```python
from build123d import *

# Parameters (mm, degrees)
F0_R     = 30.348446
F0_R_2   = 27.203675
F1_DEPTH = 15
F2_R     = 53.512853
F3_DEPTH = 18
F4_DEPTH = 81.4
F5_SIZE  = 5


with BuildPart() as f1:
    # F0 (on Top) → F1 (new body)
    with BuildSketch(Plane.XY):
        Circle(F0_R)
        Circle(F0_R_2, mode=Mode.SUBTRACT)
    extrude(amount=F1_DEPTH)

    # F2 (on face) → F3 (join)
    with BuildSketch(Plane.XY.offset(15)):
        Circle(F2_R)
    extrude(amount=F3_DEPTH)

    # F0 (on Top) → F4 (cut)
    with BuildSketch(Plane.XY):
        Circle(F0_R_2)
    extrude(amount=F4_DEPTH, mode=Mode.SUBTRACT)

    # F5
    f5_edges = [f1.edges().sort_by_distance(p)[0] for p in [
        (-53.512853, 0, 15),
    ]]
    chamfer(f5_edges, length=F5_SIZE)


solid = f1.part
```
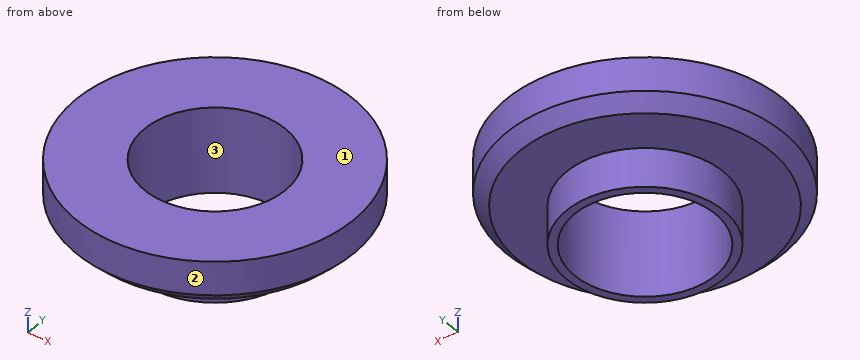
Geometry: final body of the model. Coordinates: model frame, mm. Face numbers are marked on the shaded views. Round coordinates to 2 decimals unless told otherwise and drop trailing zeros. Write each loop counter-clockwise with the first axis right and the second up, starting at its lowest first coordinate (ties: lowest second). Pieces come first, ordered by that corner, then holes. Notation, with made-up numbers: (-28, -33.75) -> (8, -33.75) arc R12 ccw to (8, -13.75) -> close; hole circle Ø1 at (89.25, 33.25). An arc over 180 degrees is marked (long way). Return JSON: item names as keys, results as strings.
Q1. Mould query, pull axis Y, two halves, no side actions, for the marked faces 1, 2 and 3. Classes: +Y half, -Y half, draft (parallel to the pull), parting line (faces both ways), or undercut.
From the geometry:
{"face 1": "draft", "face 2": "parting line", "face 3": "undercut"}
Q2. Section A-A on x = 0. Return the cut outline in (y, z).
From the geometry:
{"outline": "(-53.51, 20) -> (-48.51, 15) -> (-30.35, 15) -> (-30.35, 0) -> (-27.2, 0) -> (-27.2, 33) -> (-53.51, 33) -> close; (27.2, 0) -> (30.35, 0) -> (30.35, 15) -> (48.51, 15) -> (53.51, 20) -> (53.51, 33) -> (27.2, 33) -> close"}
Q3. Ray query, line 1 (Y direction, x = 0, z = 26); line 2 (Z direction, x = -8, y = -42.5); line 3 (X direction, y = 11.5, z = 10). Return the intervals inside material, ascending.
From the geometry:
{"line 1": "-53.51 to -27.2, 27.2 to 53.51", "line 2": "15 to 33", "line 3": "-28.09 to -24.65, 24.65 to 28.09"}
Q4. Section C-C on z = 11. Return the cut outline in (x, y), and give its area (3 significant figures).
From the geometry:
{"outline": "circle Ø60.7 at (0, 0); hole circle Ø54.41 at (0, 0)", "area": "569 mm2"}
Q5. First-contact query: pin 1 Ø5 at (x, z) = (-42, 28) entering from -Y; pin 2 Ø1.5 at (x, z) = (41, 24) entering from -Y; pin 3 Ø12 at (x, z) = (-5, 16) entering from -Y. Flat tips, straight axial feed; report the tip coordinate or a pass-through.
From the geometry:
{"pin 1": "y = -36.1", "pin 2": "y = -35.26", "pin 3": "y = -53.51"}
Q6. Section D-D on z = 31. Return the cut outline in (x, y).
From the geometry:
{"outline": "circle Ø107.03 at (0, 0); hole circle Ø54.41 at (0, 0)"}
